Source: CAD feature listing. Evaluate the final solid. Frame: model axes, mm. A direction names the side the tool comes from. Coordinates: 2 decimals unless noted, no trailing zeros. Order: outer loops, then holes, each group sorted by start corner. A loop starts at its lowest first (then second) coordinate and runs counter-clockwise, first axis right, second up.
```python
from build123d import *

# Parameters (mm, degrees)
F0_R     = 93.5
F0_R_2   = 5.5
F0_R_3   = 4.2
F0_R_4   = 71.5
F1_DEPTH = 16
F0_R_5   = 67.5
F0_R_6   = 40
F2_DEPTH = 29
F3_DEPTH = 16
F4_R     = 15.99999
F0_R_7   = 5.6
F5_DEPTH = 15


# Not quite as in the source:
# - a fillet or chamfer is up to 0.001 mm smaller than in the source, because OpenCascade refuses the exact size


with BuildPart() as f1:
    # F0 (on Top) → F1 (new body)
    with BuildSketch(Plane.XY):
        Circle(F0_R)
        with Locations((-40.75, -70.5810704084)):
            Circle(F0_R_2, mode=Mode.SUBTRACT)
        with Locations((-70.5181, -40.85)):
            Circle(F0_R_3, mode=Mode.SUBTRACT)
        with Locations((-81.5, 0)):
            Circle(F0_R_2, mode=Mode.SUBTRACT)
        Circle(F0_R_4, mode=Mode.SUBTRACT)
        with Locations((40.75, -70.5810704084)):
            Circle(F0_R_2, mode=Mode.SUBTRACT)
        with Locations((81.5, 0)):
            Circle(F0_R_2, mode=Mode.SUBTRACT)
        with Locations((-40.75, 70.5810704084)):
            Circle(F0_R_2, mode=Mode.SUBTRACT)
        with Locations((70.5181, 40.75)):
            Circle(F0_R_3, mode=Mode.SUBTRACT)
        with Locations((40.75, 70.5810704084)):
            Circle(F0_R_2, mode=Mode.SUBTRACT)
    extrude(amount=F1_DEPTH)

    # F0 (on Top) → F2 (join)
    with BuildSketch(Plane.XY):
        Circle(F0_R_4)
        Circle(F0_R_5, mode=Mode.SUBTRACT)
        Circle(F0_R_5)
        Circle(F0_R_6, mode=Mode.SUBTRACT)
    extrude(amount=F2_DEPTH)

    # F0 (on Top) → F3 (join)
    with BuildSketch(Plane.XY):
        Circle(F0_R_5)
        Circle(F0_R_6, mode=Mode.SUBTRACT)
    extrude(amount=-F3_DEPTH)

    # F4 (radius 16 in the source; OpenCascade refuses exactly that, so slightly less here)
    f4_edges = [f1.edges().sort_by_distance(p)[0] for p in [
        (-67.5, 0, -16),
    ]]
    fillet(f4_edges, radius=F4_R)

    # F0 (on Top) → F5 (join)
    with BuildSketch(Plane.XY):
        Circle(F0_R_6)
        Circle(F0_R_7, mode=Mode.SUBTRACT)
    extrude(amount=-F5_DEPTH)

    # F6 (on Front) → F7 (revolve, cut)
    with BuildSketch(Plane.XZ):
        Polygon((0, 29.0000022426), (0, 8.0000022426), (58.5, 8.0000022426), (63.5, 29.0000022426), align=None)
    revolve(axis=Axis((0, 0, 18.5000022426), (0, 0, 1)), mode=Mode.SUBTRACT)

    # F8 (on Front) → F9 (revolve, cut)
    with BuildSketch(Plane.XZ):
        Polygon((44.5, -6.9999977574), (51.4999961092, -1.4999977574), (58.5, 8.0000022426), (0, 8.0000022426), (0, -1.4999977574), (0, -6.9999977574), align=None)
    revolve(axis=Axis((0, 0, 3.2500022426), (0, 0, 1)), mode=Mode.SUBTRACT)


solid = f1.part
```
1. Section query D-D on z = -4.5. Return loops of the section in (x, y).
Findings:
outline: circle Ø133.71 at (0, 0); hole circle Ø95.36 at (0, 0)
2. Section query C-C on x = -81.5. Return loops of the section in (y, z), plus the area to 3 significant figures.
Findings:
outline: (-45.83, 0) - (-5.5, 0) - (-5.5, 16) - (-45.83, 16) - close; (5.5, 0) - (45.83, 0) - (45.83, 16) - (5.5, 16) - close
area: 1,290 mm2
3. Draft query along X for faces 4 (the face through (-52.7, 48.32, 22.41)), 5 (the face through (1, -9, -7)), 6 (the face through (0, 64, 29)). Return one class per face: released by +X, released by -X, zero draft, split by the parting line, or undercut.
Findings:
face 4: split by the parting line
face 5: undercut
face 6: zero draft
4. Section query B-B on y = 0. Count the separate pieces of the cut face and the enclosed holes in it, plus the area to 3 significant figures.
Findings:
separate pieces: 4
enclosed holes: 0
area: 2,240 mm2
5. Ray query, line 1 (Y direction, x = 40.75, z = 7.25); line 2 (Y direction, x = -40, z = 6); line 3 (X direction, y = 40, z = 10). Return the intervals inside material, ascending.
Findings:
line 1: y = -84.15 to -76.08, -65.08 to -41.2, 41.2 to 65.08, 76.08 to 84.15
line 2: y = -84.51 to -76.03, -65.13 to -40.64, 40.64 to 65.13, 76.03 to 84.51
line 3: x = -84.51 to -43.34, 43.34 to 66.39, 74.65 to 84.51
6. Access query for faces 1 (the face through (36.39, 67.23, 7.89)), 2 (the face through (-35, 63, 16)), 3 (the face through (-8.67, -39.05, -15.49)). Directions: +Z, -Z, +X, -X, +Y, -Y. A direction counts if a zero-diameter tool reaches every point of the face in a straight line with its end or side. Return the directions, or none.
Findings:
face 1: +Z, -Z
face 2: +Z
face 3: -Z
7. Pin query (flat end, axial travel): P1, Ø6, axis at x = 42, z = 5.5, coming from the +Y side; P2, Ø3, axis at x = -23, y = 24.5, coming from the -Z side; P3, Ø14.5, axis at x = -81.5, y = 0, coming from the +Z side; P4, Ø7.5, axis at x = -70.52, y = -40.85, coming from the -Z side. Return the tip coordinate at first contact, or that it passes through.
Findings:
P1: stops at y = 84.98
P2: stops at z = -15
P3: stops at z = 16
P4: passes through
